from build123d import *

# Parameters (mm, degrees)
SKETCH1_W           = 186
SKETCH1_H           = 100
BOSS_EXTRUDE1_DEPTH = 3
SKETCH2_W           = 74
SKETCH2_H           = 74
SKETCH2_R           = 1.85
CUT_EXTRUDE1_DEPTH  = 4


with BuildPart() as part:
    # Sketch1 → Boss-Extrude1 (new body)
    with BuildSketch(Plane.XY):
        with Locations((93, 50)):
            Rectangle(SKETCH1_W, SKETCH1_H)
    extrude(amount=BOSS_EXTRUDE1_DEPTH)

    # Sketch2 → Cut-Extrude1 (cut, through all)
    with BuildSketch(Plane(origin=(0, 0, 0), x_dir=(-1, 0, 0), z_dir=(0, 0, -1))):
        with Locations((-128, 47)):
            Rectangle(SKETCH2_W, SKETCH2_H)
        with Locations((-180, 7)):
            Circle(SKETCH2_R)
        with Locations((-180, 93)):
            Circle(SKETCH2_R)
        with Locations((-6, 7)):
            Circle(SKETCH2_R)
        with Locations((-6, 93)):
            Circle(SKETCH2_R)
    extrude(amount=-CUT_EXTRUDE1_DEPTH, mode=Mode.SUBTRACT)


solid = part.part
Verification items for the finished model (mm, model axes). Give positions to 0.01 mm unless a question says otherwise; leave off trailing zeros. Loops run counter-clockwise (first coordinate to the right, second up) from the corner with the lowest first, then second, coordinate; pieces in that order, holes last. Notation, with made-up numbers: (83, -28) - (141, -28) arc R17 cw to (141, -10) - close; hole circle Ø8 at (-7, 26.5). An arc over 180 degrees is marked (long way). Write each question's results on one line, items separated by ' | '.
1) Material ranges on L1, parallel to Y at x = 6, z = 1.3; L2, parallel to X at y = 93, z = 2.2; L3, parallel to X at y = 50.5, z = 1.95, recorded low to high. Write a range as from..to.
Solution:
L1: 0..5.15, 8.85..91.15, 94.85..100 | L2: 0..4.15, 7.85..178.15, 181.85..186 | L3: 0..91, 165..186
2) Sectioned sample at D-D on z = 0.6. Record the boundary of the cut face in (x, y).
Solution:
outline: (0, 0) - (186, 0) - (186, 100) - (0, 100) - close; hole circle Ø3.7 at (6, 7); hole circle Ø3.7 at (6, 93); hole (91, 10) - (165, 10) - (165, 84) - (91, 84) - close; hole circle Ø3.7 at (180, 7); hole circle Ø3.7 at (180, 93)
3) Sectioned sample at C-C on x = 153. Record the boundary of the cut face in (y, z), plus the area to 3 significant figures.
Solution:
outline: (0, 0) - (10, 0) - (10, 3) - (0, 3) - close; (84, 0) - (100, 0) - (100, 3) - (84, 3) - close | area: 78.0 mm2
4) Mould release check, pull along X, two halves, no side actions. Record for faces 1 (the flat face through (71, 51, 0)), 2 (the cylindrical face through (179.146, 91.359, 1.479)): pulls with the +X half, pulls with the -X half, needs draft (parallel to the pull), parting line crosses it, or undercut.
Solution:
face 1: needs draft | face 2: undercut
5) Sectioned sample at B-B on x = 6. Record the boundary of the cut face in (y, z), plus the area to 3 significant figures.
Solution:
outline: (0, 0) - (5.15, 0) - (5.15, 3) - (0, 3) - close; (8.85, 0) - (91.15, 0) - (91.15, 3) - (8.85, 3) - close; (94.85, 0) - (100, 0) - (100, 3) - (94.85, 3) - close | area: 278 mm2
6) Sectioned sample at A-A on y = 7. Record the boundary of the cut face in (x, z), plus the area to 3 significant figures.
Solution:
outline: (0, 0) - (4.15, 0) - (4.15, 3) - (0, 3) - close; (7.85, 0) - (178.15, 0) - (178.15, 3) - (7.85, 3) - close; (181.85, 0) - (186, 0) - (186, 3) - (181.85, 3) - close | area: 536 mm2
